from build123d import *

# Parameters (mm, degrees)
F0_W      = 40
F0_H      = 40
F0_R      = 8
F1_DEPTH  = 40
F2_W      = 21
F2_H      = 21
F3_DEPTH  = 30
F5_R      = 5
F6_DEPTH  = 11
F7_R      = 6.3
F8_DEPTH  = 8
F9_R      = 7
F10_DEPTH = 5
F11_R     = 5
F12_SIZE  = 1
F13_R     = 1.25
F14_DEPTH = 10


with BuildPart() as f1:
    # F0 (on Top) → F1 (new body)
    with BuildSketch(Plane.XY):
        Rectangle(F0_W, F0_H)
        Circle(F0_R, mode=Mode.SUBTRACT)
    extrude(amount=F1_DEPTH)


with BuildPart() as f3:
    # F2 (on Top) → F3 (new body)
    with BuildSketch(Plane.XY):
        Rectangle(F2_W, F2_H)
    extrude(amount=F3_DEPTH)


with BuildPart() as f1_1:
    add(f1.part)

    # F4: cut F3
    add(f3.part, mode=Mode.SUBTRACT)

    # F5 (on face) → F6 (cut)
    with BuildSketch(Plane.YZ.offset(20)):
        with Locations((0, 20)):
            Circle(F5_R)
    extrude(amount=-F6_DEPTH, mode=Mode.SUBTRACT)

    # F7 (on face) → F8 (cut)
    with BuildSketch(Plane.YZ.offset(20)):
        with Locations((0, 20)):
            Circle(F7_R)
    extrude(amount=-F8_DEPTH, mode=Mode.SUBTRACT)

    # F9 (on face) → F10 (cut)
    with BuildSketch(Plane.YZ.offset(20)):
        with Locations((0, 20)):
            Circle(F9_R)
    extrude(amount=-F10_DEPTH, mode=Mode.SUBTRACT)

    # F11
    f11_edges = [f1_1.edges().sort_by_distance(p)[0] for p in [
        (20, 20, 20),
        (-20, 20, 20),
        (-20, -20, 20),
        (20, -20, 20),
    ]]
    fillet(f11_edges, radius=F11_R)

    # F12
    f12_edges = [f1_1.edges().sort_by_distance(p)[0] for p in [
        (-8, 0, 40),
    ]]
    chamfer(f12_edges, length=F12_SIZE)

    # F13 (on face) → F14 (cut)
    with BuildSketch(Plane.XY.offset(40)):
        with Locations((-15, 15)):
            Circle(F13_R)
        with Locations((-15, -15)):
            Circle(F13_R)
        with Locations((15, -15)):
            Circle(F13_R)
        with Locations((15, 15)):
            Circle(F13_R)
    extrude(amount=-F14_DEPTH, mode=Mode.SUBTRACT)


solid = f1_1.part
Check sheet for the modelled part. Datum: model origin and axes. Units: mm. A direction names the side the tool comes from. Round coordinates to 2 decimals unless told otherwise and drop trailing zeros. Loops run counter-clockwise (first coordinate to the right, second up) from the corner with the lowest first, then second, coordinate; pieces in that order, holes last. Notation, with made-up numbers: (49, 50.25) -> (105, 50.25) arc R22 cw to (105, 81.25) -> close; hole circle Ø9 at (-11.5, -5). An arc over 180 degrees is marked (long way). Put each result on its own line as item: value. Start each with the question number.
1. Section check A-A (x = 0). Enter the section's corners in (y, z).
2. Section check B-B (y = 0). Enter the section's corners in (x, z), plus the area to 3 significant figures.
3. Draft check along X on faces 1 (the face through (14.079, 15.845, 35.07)), 2 (the face through (-19, -18, 20)), 3 (the face through (0, 20, 20)). Enter one of: +X half, -X half, draft (parallel to the pull), parting line (faces both ways), or undercut.
4. Scan lines: probe 1 along X at (y, z) = (9.5, 10); probe 2 along Z at (x, y) = (16.3, 0). Record each from-to range of solid material in increasing order.
5. Section check D-D (z = 23). Enter the section's corners in (x, y).
6. Access from +Z, -Z, +X, -X, +Y, -Y to the whole of each face (thin tool, end or side, straight path). Record for faces 4 (the face through (13.521, -0.82, 26.246)), 5 (the face through (14.84, -13.76, 35.07)), 6 (the face through (0, -10.5, 15)).
7. Section check C-C (z = 8). Enter the section's corners in (x, y).
8. Gauge pin test, flat ends, axial feed: pin 1 (1.5 mm diameter, centred on x = 15, y = 15, fed in from +Z); pin 2 (9.5 mm diameter, centred on x = 0, y = 0, fed in from +Z). Record the tip position at first contact, or that the pin passes through.
Findings:
1. outline: (-20, 0) -> (-10.5, 0) -> (-10.5, 30) -> (-8, 30) -> (-8, 39) -> (-9, 40) -> (-20, 40) -> close; (8, 30) -> (10.5, 30) -> (10.5, 0) -> (20, 0) -> (20, 40) -> (9, 40) -> (8, 39) -> close
2. outline: (-20, 0) -> (-10.5, 0) -> (-10.5, 30) -> (-8, 30) -> (-8, 39) -> (-9, 40) -> (-20, 40) -> close; (8, 30) -> (10.5, 30) -> (10.5, 25) -> (12, 25) -> (12, 26.3) -> (15, 26.3) -> (15, 27) -> (20, 27) -> (20, 40) -> (9, 40) -> (8, 39) -> close; (10.5, 0) -> (20, 0) -> (20, 13) -> (15, 13) -> (15, 13.7) -> (12, 13.7) -> (12, 15) -> (10.5, 15) -> close
2. area: 686 mm^2
3. face 1: undercut
3. face 2: -X half
3. face 3: draft
4. probe 1: x = -20 to -10.5, 10.5 to 20
4. probe 2: z = 0 to 13, 27 to 40
5. outline: (-20, -15) arc R5 ccw to (-15, -20) -> (15, -20) arc R5 ccw to (20, -15) -> (20, -6.32) -> (15, -6.32) -> (15, -5.54) -> (12, -5.54) -> (12, -4) -> (10.5, -4) -> (10.5, -10.5) -> (-10.5, -10.5) -> (-10.5, 10.5) -> (10.5, 10.5) -> (10.5, 4) -> (12, 4) -> (12, 5.54) -> (15, 5.54) -> (15, 6.32) -> (20, 6.32) -> (20, 15) arc R5 ccw to (15, 20) -> (-15, 20) arc R5 ccw to (-20, 15) -> close
6. face 4: +X
6. face 5: +Z
6. face 6: -Z
7. outline: (-20, -15) arc R5 ccw to (-15, -20) -> (15, -20) arc R5 ccw to (20, -15) -> (20, 15) arc R5 ccw to (15, 20) -> (-15, 20) arc R5 ccw to (-20, 15) -> close; hole (-10.5, -10.5) -> (10.5, -10.5) -> (10.5, 10.5) -> (-10.5, 10.5) -> close
8. pin 1: stops at z = 30
8. pin 2: passes through
